The model under review builds one solid part; all positions refer to its coordinate system, in mm. Face numbers are marked on the shaded views. A direction names the side the tool comes from. Coordinates: 2 decimals unless noted, no trailing zeros. Write each loop counter-clockwise with the first axis right and the second up, starting at its lowest first coordinate (ties: lowest second). Pieces come first, ordered by that corner, then holes. Notation, with made-up numbers: (60, 32) - (105, 32) arc R17 ccw to (105, 51) - close; hole circle Ø7 at (7, -31). An arc over 180 degrees is marked (long way). Put each result on its own line as item: value.
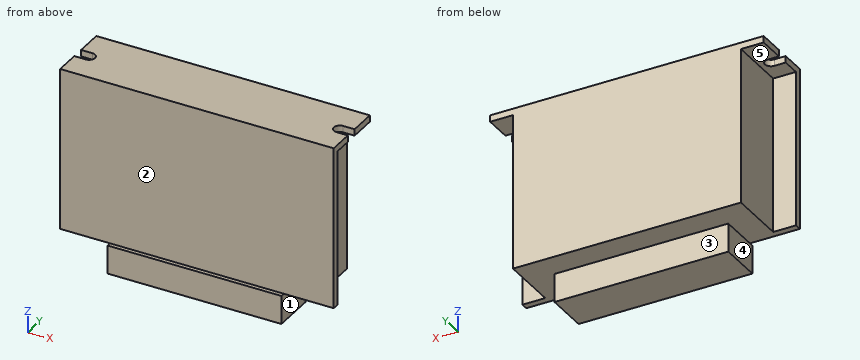
from build123d import *

# Parameters (mm, degrees)
SKETCH_1_W          = 96
SKETCH_1_H          = 57
EXTRUDE_1_DEPTH     = 22.5
SKETCH_2_W          = 61
SKETCH_2_H          = 15
EXTRUDE_2_DEPTH     = 10
SKETCH_3_W          = 8
SKETCH_3_H          = 54.7
CUT_EXTRUDE_1_DEPTH = 20.1
CUT_EXTRUDE_2_DEPTH = 84.64412711


with BuildPart() as part:
    # 草图1 → 凸台-拉伸1 (new body)
    with BuildSketch(Plane(origin=(0, 0, 0), x_dir=(1, 0, 0), z_dir=(0, 1, 0))):
        Rectangle(SKETCH_1_W, SKETCH_1_H)
    extrude(amount=EXTRUDE_1_DEPTH)

    # 草图2 → 凸台-拉伸2 (add)
    with BuildSketch(Plane(origin=(0, 0, -28.5), x_dir=(-1, 0, 0), z_dir=(0, 0, -1))):
        with Locations((0, 6)):
            Rectangle(SKETCH_2_W, SKETCH_2_H)
    extrude(amount=EXTRUDE_2_DEPTH)

    # 草图3 → 切除-拉伸1 (cut)
    with BuildSketch(Plane(origin=(0, 22.5, 0), x_dir=(1, 0, 0), z_dir=(0, 1, 0))):
        with Locations((44, 1.15)):
            Rectangle(SKETCH_3_W, SKETCH_3_H)
    cut_extrude_1 = extrude(amount=-CUT_EXTRUDE_1_DEPTH, mode=Mode.SUBTRACT)

    # 草图4 → 切除-拉伸2 (cut, through all)
    with BuildSketch(Plane(origin=(0, 0, 26.2), x_dir=(-1, 0, 0), z_dir=(0, 0, -1))):
        with BuildLine():
            Line((-44, 8.8), (-48, 8.8))
            Line((-48, 8.8), (-48, 13))
            Line((-48, 13), (-44, 13))
            ThreePointArc((-44, 13), (-41.9, 10.9), (-44, 8.8))
        make_face()
    cut_extrude_2 = extrude(amount=-CUT_EXTRUDE_2_DEPTH, mode=Mode.SUBTRACT)

    # 镜向2: 切除-拉伸1, 切除-拉伸2 across plane
    add(cut_extrude_1.mirror(Plane(origin=(0, 0, 0), x_dir=(0, 0, 1), z_dir=(1, 0, 0))), mode=Mode.SUBTRACT)
    add(cut_extrude_2.mirror(Plane(origin=(0, 0, 0), x_dir=(0, 0, 1), z_dir=(1, 0, 0))), mode=Mode.SUBTRACT)


solid = part.part
1. For pin 1 Ø4 at (x, z) = (-43.5, -1.5) entering from +Y; pin 2 Ø8 at (y, z) = (5, -33) entering from -X; pin 3 Ø3 at (x, y) = (-24, 19.5) entering from -Z, all flat-tipped, find the tip position at first contact; note any pin that passes through.
Determined:
pin 1: stops at y = 2.4
pin 2: stops at x = -30.5
pin 3: stops at z = -28.5
2. Machinability: for the marked faces 1, 2, 3, 4 and 5, which of the approach directions +Z, -Z, +X, -X, +Y, -Y give a long, thin tool a straight path to every point of the face, cutting with its end or side? Answer none if there is none.
Determined:
face 1: -Z, +X, +Y, -Y
face 2: +Z, +X, -X, -Y
face 3: -Z, +X, -X, +Y
face 4: -Z, -X, +Y, -Y
face 5: -Z, -X, +Y
3. To check wall thickness, follow probe 1 along Y at (x, z) = (-31.5, 21.5); probe 2 along X at (y, z) = (18.75, 20); probe 3 along Z at (x, y) = (15.5, 14). State the ranges of each line that lie inside material, in increasing order.
Determined:
probe 1: y = 0 to 22.5
probe 2: x = -40 to 40
probe 3: z = -28.5 to 28.5
4. Consider section B-B on y = 10.9. State the section outline as (x, z) points.
Determined:
outline: (-41.9, 26.2) - (-40, 26.2) - (-40, -28.5) - (-30.5, -28.5) - (-30.5, -38.5) - (30.5, -38.5) - (30.5, -28.5) - (40, -28.5) - (40, 26.2) - (41.9, 26.2) - (41.9, 28.5) - (-41.9, 28.5) - close
5. Consider section C-C on x = 15.5. State the section outline as (y, z) points, plus the area to 3 significant figures.
Determined:
outline: (-1.5, -38.5) - (13.5, -38.5) - (13.5, -28.5) - (22.5, -28.5) - (22.5, 28.5) - (0, 28.5) - (0, -28.5) - (-1.5, -28.5) - close
area: 1,430 mm^2
6. Consider section A-A on z = -19. State the section outline as (x, y) points, plus the area to 3 significant figures.
Determined:
outline: (-48, 0) - (48, 0) - (48, 2.4) - (40, 2.4) - (40, 22.5) - (-40, 22.5) - (-40, 2.4) - (-48, 2.4) - close
area: 1,840 mm^2
7. Consider section D-D on z = -31.5. State the section outline as (x, y) points, plus the area to 3 significant figures.
Determined:
outline: (-30.5, -1.5) - (30.5, -1.5) - (30.5, 13.5) - (-30.5, 13.5) - close
area: 915 mm^2
